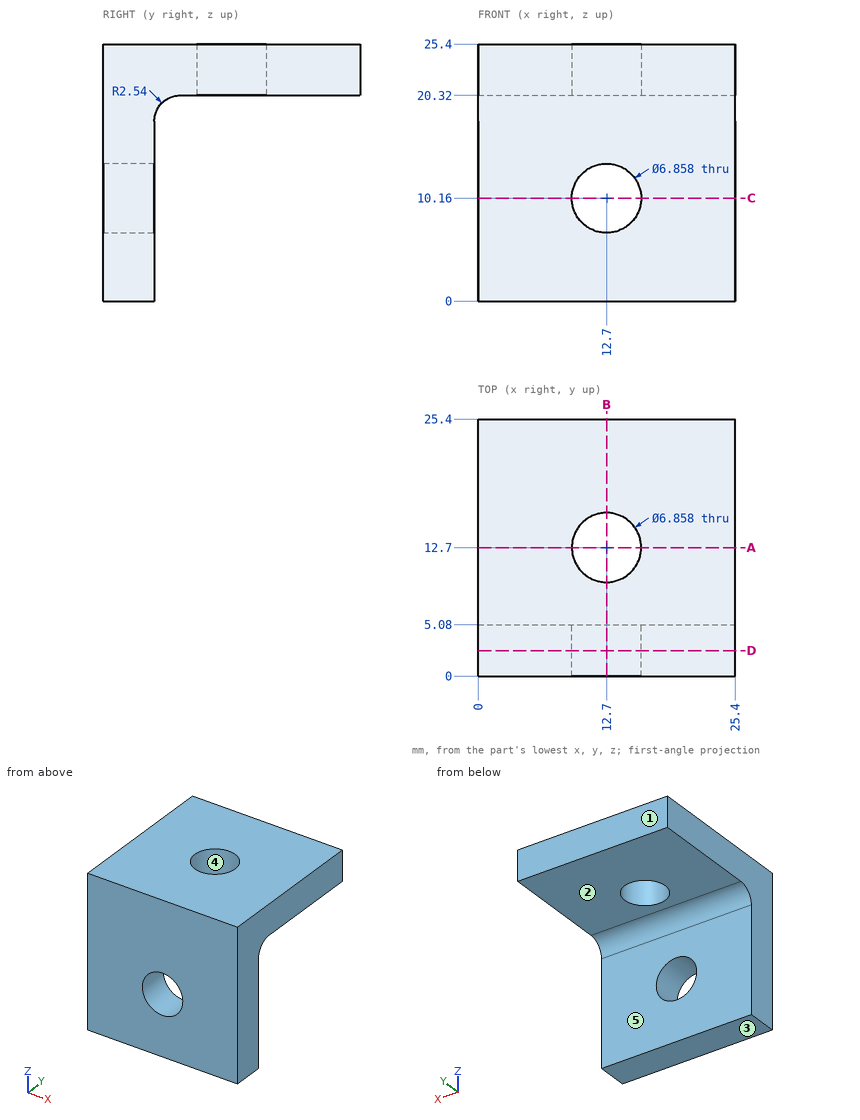
The drawing under review shows one solid part. Ordinate dimensions are in mm from its lowest x, y, z. A direction names the side the tool comes from. Coordinates: 2 decimals unless noted, no trailing zeros. Order: outer loops, then holes, each group sorted by start corner. A loop starts at its lowest first (then second) coordinate and runs counter-clockwise, first axis right, second up. Notation, with made-up numbers: (-25.75, 11.25) -> (-5.75, 11.25) arc R12 cw to (-5.75, 33.25) -> close; hole circle Ø5 at (73.25, 71.25). An arc over 180 degrees is marked (long way). Answer in a Markdown table with one row per item. Add a question column.
Item 1: We need section B-B on x = 12.7. Write out the cut boundary in (y, z), plus the area to 3 significant figures.
Item 2: To check wall thickness, follow probe 1 along X at (y, z) = (1.75, 10.16); probe 2 along Z at (x, y) = (21.75, 10.5). State the ranges of each line that lie inside material, in increasing order.
Item 3: Clearance check with flat-ended pins moving along their axes: pin 1 (14 mm diameter, centred on x = 7.5, y = 14.5, fed in from -Z); pin 2 (4 mm diameter, centred on x = 8, z = 14, fed in from +Y). State where each tip first meets the part, or that it passes through.
Item 4: Mouldability with a two-part tool opening along Y and no side actions: class the marked faces 3, 4 and 5 as +Y half, -Y half, draft (parallel to the pull), parting line (faces both ways), or undercut.
Item 5: We need section A-A on y = 12.7. Write out the cut boundary in (x, z).
Item 6: We need section D-D on y = 2.5. Write out the cut boundary in (x, z), plus the area to 3 significant figures.
Item 7: Machinability: for the marked faces 1 and 2, which of the approach directions +Z, -Z, +X, -X, +Y, -Y give a long, thin tool a straight path to every point of the face, cutting with its end or side? Answer none if there is none.
Item 8: We need section C-C on z = 10.16. Write out the cut boundary in (x, y), plus the area to 3 significant figures.
Final values:
| question | item | result |
|---|---|---|
| 1 | outline | (0, 0) -> (5.08, 0) -> (5.08, 6.73) -> (0, 6.73) -> close; (0, 13.59) -> (5.08, 13.59) -> (5.08, 17.78) arc R2.54 cw to (7.62, 20.32) -> (9.27, 20.32) -> (9.27, 25.4) -> (0, 25.4) -> close; (16.13, 20.32) -> (25.4, 20.32) -> (25.4, 25.4) -> (16.13, 25.4) -> close |
| 1 | area | 164 mm2 |
| 2 | probe 1 | x = 0 to 9.27, 16.13 to 25.4 |
| 2 | probe 2 | z = 20.32 to 25.4 |
| 3 | pin 1 | stops at z = 20.32 |
| 3 | pin 2 | stops at y = 5.08 |
| 4 | face 3 | draft |
| 4 | face 4 | undercut |
| 4 | face 5 | +Y half |
| 5 | outline | (0, 20.32) -> (9.27, 20.32) -> (9.27, 25.4) -> (0, 25.4) -> close; (16.13, 20.32) -> (25.4, 20.32) -> (25.4, 25.4) -> (16.13, 25.4) -> close |
| 6 | outline | (0, 0) -> (25.4, 0) -> (25.4, 25.4) -> (0, 25.4) -> close; hole circle Ø6.86 at (12.7, 10.16) |
| 6 | area | 608 mm2 |
| 7 | face 1 | +Z, -Z, +X, -X, +Y |
| 7 | face 2 | -Z, +X, -X, +Y |
| 8 | outline | (0, 0) -> (9.27, 0) -> (9.27, 5.08) -> (0, 5.08) -> close; (16.13, 0) -> (25.4, 0) -> (25.4, 5.08) -> (16.13, 5.08) -> close |
| 8 | area | 94.2 mm2 |
